Work out the finished part from the listing and answer in its coordinate system (mm). Give positions to 0.01 mm unless a question says otherwise; leave off trailing zeros. Order: outer loops, then holes, each group sorted by start corner. A loop starts at its lowest first (then second) coordinate and runs counter-clockwise, first axis right, second up. Notation, with made-up numbers: (33.25, -0.5) - (76.25, -0.5) arc R13 ccw to (76.25, 23.5) - close; hole circle Ø7 at (-16, 10.5). An arc over 180 degrees is marked (long way). Write each question's results on one line, items separated by ' | '.
from build123d import *

# Parameters (mm, degrees)
SKETCH_1_R      = 5
EXTRUDE_1_DEPTH = 4


with BuildPart() as part:
    # 草图1 → 凸台-拉伸1 (new body)
    with BuildSketch(Plane.XY):
        with BuildLine():
            Line((-5.5, 135.520010959), (-5.5, 12.479983974))
            ThreePointArc((-5.5, 12.479983974), (-6.05722499, 8.429521038), (-7.6875, 4.67999399))
            ThreePointArc((-7.6875, 4.67999399), (-7.870390208, -4.365427582), (-0.099998457, -8.999444444))
            Line((-0.099998457, -8.999444444), (0.099998457, -8.999444444))
            ThreePointArc((0.099998457, -8.999444444), (7.870390208, -4.365427582), (7.6875, 4.67999399))
            ThreePointArc((7.6875, 4.67999399), (6.05722499, 8.429521038), (5.5, 12.479983974))
            Line((5.5, 12.479983974), (5.5, 135.520016026))
            ThreePointArc((5.5, 135.520016026), (6.05722499, 139.570478962), (7.6875, 143.32000601))
            ThreePointArc((7.6875, 143.32000601), (7.870390208, 152.365427582), (0.099998457, 156.999444444))
            Line((0.099998457, 156.999444444), (-0.099998457, 156.999444444))
            ThreePointArc((-0.099998457, 156.999444444), (-7.870390208, 152.365427582), (-7.6875, 143.32000601))
            ThreePointArc((-7.6875, 143.32000601), (-6.057224306, 139.570476523), (-5.5, 135.520010959))
        make_face()
        Circle(SKETCH_1_R, mode=Mode.SUBTRACT)
        with Locations((0, 148)):
            Circle(SKETCH_1_R, mode=Mode.SUBTRACT)
    extrude(amount=EXTRUDE_1_DEPTH)


solid = part.part
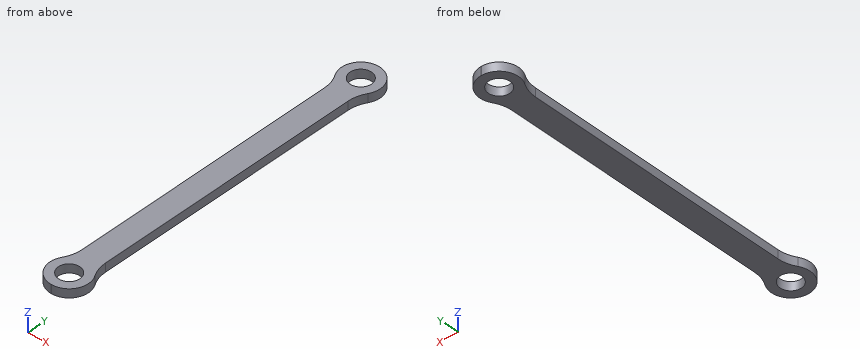
1. Straight lines are drawn through the part: line 1 (Y direction, x = 0, z = 2.65); line 2 (Y direction, x = 2, z = 3.8); line 3 (Y direction, x = 7.5, z = 2.7). For each, find the intervals that lie inside material, in ascending order. Write a range as [from, to].
Answer list:
line 1: [-9, -5], [5, 143], [153, 157] | line 2: [-8.77, -4.58], [4.58, 143.42], [152.58, 156.77] | line 3: [-4.97, 5], [143, 152.97]
2. A cutting plane is placed at A-A, the plane y = 0. Write down the section's boundary in (x, z).
Answer list:
outline: (-9, 0) - (-5, 0) - (-5, 4) - (-9, 4) - close; (5, 0) - (9, 0) - (9, 4) - (5, 4) - close
3. A cutting plane is placed at C-C, the plane x = 3.25. Write down the section's boundary in (y, z).
Answer list:
outline: (-8.39, 0) - (-3.8, 0) - (-3.8, 4) - (-8.39, 4) - close; (3.8, 0) - (144.2, 0) - (144.2, 4) - (3.8, 4) - close; (151.8, 0) - (156.39, 0) - (156.39, 4) - (151.8, 4) - close
4. A cutting plane is placed at D-D, the plane y = 45. Write down the section's boundary in (x, z), then the cut area to 3 significant figures.
Answer list:
outline: (-5.5, 0) - (5.5, 0) - (5.5, 4) - (-5.5, 4) - close | area: 44.0 mm^2
5. Given P1, Ø1.2, axis at y = 71, z = 2, coming from the +X side; P2, Ø1, axis at x = -6, z = 0.5, coming from the -Y side; P3, Ø2, axis at x = 6, z = 3.5, coming from the +Y side, each flat-ended and moving along its own axis, determine where each tip first touches the part or whether it passes through.
Answer list:
P1: x = 5.5 | P2: y = -7.12 | P3: y = 155.48
6. A cutting plane is placed at B-B, the plane z = 1.6. Write down the section's boundary in (x, y), then the cut area to 3 significant figures.
Answer list:
outline: (-7.69, 4.68) arc R9 ccw to (-0.1, -9) - (0.1, -9) arc R9 ccw to (7.69, 4.68) arc R15 cw to (5.5, 12.48) - (5.5, 135.52) arc R15 cw to (7.69, 143.32) arc R9 ccw to (0.1, 157) - (-0.1, 157) arc R9 ccw to (-7.69, 143.32) arc R15 cw to (-5.5, 135.52) - (-5.5, 12.48) arc R15 cw to start; hole circle Ø10 at (0, 0); hole circle Ø10 at (0, 148) | area: 1,810 mm^2
